Could you check a few things on this model? Use its own coordinates, in mm. A direction names the side the tool comes from. Give positions to 0.01 mm unless a question says otherwise; leave off trailing zeros. Order: outer loops, then holes, each group sorted by start corner. A loop starts at its lowest first (then second) coordinate and runs counter-clockwise, first axis right, second up. Notation, with made-up numbers: (87.5, -32.75) -> (146.5, -32.75) arc R29 cw to (146.5, 3.25) -> close; hole circle Ø1 at (49, -28). An arc over 180 degrees is marked (long way). Answer as CSV lines item,"result". Start each with the question number.
(1) On a 3-axis mill with a long thin cutter (end or side, diameter ignored), from which of +Z, -Z, +X, -X, +Y, -Y can I reach the whole of each face in a straight line? I mean faces 1 (the face through (-1.6, 0, -4.5)), 2 (the face through (-3.78, -20.36, -4.15)). Say none if no direction works.
(2) I want a section at D-D (x = -4). Please give me the cut outline in (y, z).
(3) I want a section at A-A (x = 0). Give the number of separate pieces and of enclosed holes in the cut face, plus the area to 3 significant figures.
(4) I want a section at C-C (y = -46). Please give me the cut outline in (x, z).
(5) I want a section at B-B (z = 1.5). Please give me the cut outline in (x, y), plus the area to 3 significant figures.
(6) We'd pull the mould along X, two halves only. Please class faces 3 (the face through (-3.78, -37.82, -4.15)), 4 (the face through (-0.9, -34.4, 6.8)), 5 (the face through (-1.6, -69.85, -4.5)): released by +X, released by -X, zero draft, split by the parting line, or undercut.
(7) I need wall thicknesses on L1, parallel to Y at x = 4, z = -4.25; L2, parallel to Z at x = 1.75, y = -61; L3, parallel to X at y = -18.5, z = -2.5. Which ranges of each line are inside material? Lowest first, please.
(8) Will these pins go through, and if not, where does the flat tip stop? pin 1 Ø1 at (y, z) = (-45, 4.5) entering from +X; pin 2 Ø4 at (x, y) = (3, -47.5) entering from +Z; pin 3 Ø4 at (y, z) = (-50, -5) entering from -X; pin 4 Ø7.5 at (x, z) = (0, 0) entering from +Y.
```python
from build123d import *

# Parameters (mm, degrees)
F0_R     = 6.858
F0_R_2   = 4.6228
F1_DEPTH = 69.85
F2_R     = 4.7625
F3_DEPTH = 25.4


with BuildPart() as f1:
    # F0 (on Front) → F1 (new body)
    with BuildSketch(Plane.XZ):
        Circle(F0_R)
        Circle(F0_R_2, mode=Mode.SUBTRACT)
    extrude(amount=F1_DEPTH)

    # F2 (on Top) → F3 (cut)
    with BuildSketch(Plane.XY):
        with Locations((0, -17.4625)):
            Circle(F2_R)
        with Locations((0, -34.925)):
            Circle(F2_R)
        with Locations((0, -52.3875)):
            Circle(F2_R)
    extrude(amount=-F3_DEPTH, mode=Mode.SUBTRACT)


solid = f1.part
```
Final values:
1,face 1,"+Z, -Z, +X, -X, +Y"
1,face 2,"-Z"
2,outline,"(-69.85, -5.57) -> (-54.97, -5.57) -> (-54.97, -2.32) -> (-69.85, -2.32) -> close; (-69.85, 2.32) -> (0, 2.32) -> (0, 5.57) -> (-69.85, 5.57) -> close; (-49.8, -5.57) -> (-37.51, -5.57) -> (-37.51, -2.32) -> (-49.8, -2.32) -> close; (-32.34, -5.57) -> (-20.05, -5.57) -> (-20.05, -2.32) -> (-32.34, -2.32) -> close; (-14.88, -5.57) -> (0, -5.57) -> (0, -2.32) -> (-14.88, -2.32) -> close"
3,separate pieces,"5"
3,enclosed holes,"0"
3,area,"248 mm²"
4,outline,"circle Ø13.72 at (0, 0); hole circle Ø9.25 at (0, 0)"
5,outline,"(-6.69, -69.85) -> (-4.37, -69.85) -> (-4.37, 0) -> (-6.69, 0) -> close; (4.37, -69.85) -> (6.69, -69.85) -> (6.69, 0) -> (4.37, 0) -> close"
5,area,"324 mm²"
6,face 3,"undercut"
6,face 4,"split by the parting line"
6,face 5,"zero draft"
7,L1,"-69.85 to -54.97, -49.8 to -37.51, -32.34 to -20.05, -14.88 to 0"
7,L2,"-6.63 to -4.28, 4.28 to 6.63"
7,L3,"-6.39 to -4.65, 4.65 to 6.39"
8,pin 1,"x = 5.57"
8,pin 2,"z = 6.78"
8,pin 3,"x = -6.17"
8,pin 4,"through"
